```python
from build123d import *

# Parameters (mm, degrees)
SKETCH_1_W          = 20
SKETCH_1_H          = 12
SKETCH_1_W_2        = 4.2
SKETCH_1_H_2        = 6.9
EXTRUDE_1_DEPTH     = 9.5
CUT_EXTRUDE_START   = 9.5
SKETCH_1_4_W        = 20
SKETCH_1_4_H        = 3
CUT_EXTRUDE_2_DEPTH = 1
SKETCH_1_6_W        = 8.2
SKETCH_1_6_H        = 6.9
CUT_EXTRUDE_4_DEPTH = 2
SKETCH_2_R          = 0.7
SKETCH_2_R_2        = 0.35
CUT_EXTRUDE_5_DEPTH = 26.184320519
SKETCH_2_3_R        = 1
CUT_EXTRUDE_6_DEPTH = 7.5


with BuildPart() as part:
    # 草图1 → 凸台-拉伸1 (new body)
    with BuildSketch(Plane(origin=(0, 0, 0), x_dir=(1, 0, 0), z_dir=(0, 1, 0))):
        with Locations((10, -6)):
            Rectangle(SKETCH_1_W, SKETCH_1_H)
        with Locations((8, -8.25)):
            Rectangle(SKETCH_1_W_2, SKETCH_1_H_2, mode=Mode.SUBTRACT)
    extrude(amount=EXTRUDE_1_DEPTH)

    # 草图1<4> → 切除-拉伸2 (cut)
    with BuildSketch(Plane(origin=(0, 0, 0), x_dir=(1, 0, 0), z_dir=(0, 1, 0)).offset(CUT_EXTRUDE_START)):
        with Locations((10, -8)):
            Rectangle(SKETCH_1_4_W, SKETCH_1_4_H)
    extrude(amount=-CUT_EXTRUDE_2_DEPTH, mode=Mode.SUBTRACT)

    # 草图1<6> → 切除-拉伸4 (cut)
    with BuildSketch(Plane(origin=(0, 0, 0), x_dir=(1, 0, 0), z_dir=(0, 1, 0)).offset(CUT_EXTRUDE_START)):
        with Locations((8, -8.25)):
            Rectangle(SKETCH_1_6_W, SKETCH_1_6_H)
    extrude(amount=-CUT_EXTRUDE_4_DEPTH, mode=Mode.SUBTRACT)

    # 草图2 → 切除-拉伸5 (cut, through all)
    with BuildSketch(Plane(origin=(0, 9.5, 0), x_dir=(1, 0, 0), z_dir=(0, 1, 0))):
        with Locations(Location((3, -3, 0), (0, 0, 270))):
            Circle(SKETCH_2_R)
        with Locations(Location((3, -9, 0), (0, 0, 270))):
            Circle(SKETCH_2_R)
        with Locations(Location((17, -3, 0), (0, 0, 270))):
            Circle(SKETCH_2_R)
        with Locations(Location((17, -9, 0), (0, 0, 270))):
            Circle(SKETCH_2_R)
        with Locations(Location((7, -3, 0), (0, 0, 270))):
            Circle(SKETCH_2_R_2)
        with Locations(Location((14, -3, 0), (0, 0, 270))):
            Circle(SKETCH_2_R_2)
        with Locations(Location((3, -6, 0), (0, 0, 270))):
            Circle(SKETCH_2_R_2)
        with Locations(Location((17, -6, 0), (0, 0, 270))):
            Circle(SKETCH_2_R_2)
    extrude(amount=-CUT_EXTRUDE_5_DEPTH, mode=Mode.SUBTRACT)

    # 草图2<3> → 切除-拉伸6 (cut)
    with BuildSketch(Plane(origin=(0, 9.5, 0), x_dir=(1, 0, 0), z_dir=(0, 1, 0))):
        with Locations(Location((3, -3, 0), (0, 0, 270))):
            Circle(SKETCH_2_3_R)
        with Locations(Location((3, -9, 0), (0, 0, 330))):
            Circle(SKETCH_2_3_R)
        with Locations(Location((17, -3, 0), (0, 0, 270))):
            Circle(SKETCH_2_3_R)
        with Locations(Location((17, -9, 0), (0, 0, 330))):
            Circle(SKETCH_2_3_R)
    extrude(amount=-CUT_EXTRUDE_6_DEPTH, mode=Mode.SUBTRACT)


solid = part.part
```
Input: part model. Units: mm. Frame: model coordinates. A direction names the side the tool comes from. Coordinates: 2 decimals unless noted, no trailing zeros. Write each loop counter-clockwise with the first axis right and the second up, starting at its lowest first coordinate (ties: lowest second). Pieces come first, ordered by that corner, then holes.
1) Mould query, pull axis Z, two halves, no side actions, for faces 1 (the flat face through (10, 5, 12)), 2 (the flat face through (20, 5, 6)), 3 (the flat face through (1, 8.5, 8)). Classes: pulls with the +Z half, pulls with the -Z half, needs draft (parallel to the pull), parting line crosses it, or undercut.
2) Material intervals for line 1 along X through (y, z) = (0.8, 9); line 2 along X through (y, z) = (7.75, 9); line 3 along X through (y, z) = (7, 9), sorted ascending.
3) Section D-D on z = 9. Output: boundary loops of the cut face in (x, y), and give its area (3 significant figures).
4) Section A-A on z = 11.25. Output: boundary loops of the cut face in (x, y), and give its area (3 significant figures).
5) Pin query (flat end, axial travel): pin 1 Ø1.5 at (x, z) = (11.5, 7) entering from -Y; pin 2 Ø1 at (x, z) = (11, 6.5) entering from +Y. Return the tip coordinate at first contact, or that it passes through.
6) Set-up query: faces 4 (the flat face through (0, 5, 6)), 5 (the flat face through (10.1, 4, 8)), 6 (the flat face through (1, 9, 9.5)), 7 (the cylindrical face through (2.324, 5.802, 9.737)). Return all of +Z, -Z, +X, -X, +Y, -Y with unobstructed straight access to the full face (end or side cutting, diameter ignored); none if empty.
7) Section B-B on x = 6.25. Output: boundary loops of the cut face in (y, z).
8) Section C-C on y = 4.75. State how many separate pieces and enclosed holes the cut face has, and give its area (3 significant figures).
Check result:
1. face 1: pulls with the +Z half
1. face 2: needs draft
1. face 3: undercut
2. line 1: x = 0 to 2.3, 3.7 to 5.9, 10.1 to 16.3, 17.7 to 20
2. line 2: x = 0 to 2, 12.1 to 16, 18 to 20
2. line 3: x = 0 to 2, 4 to 5.9, 10.1 to 16, 18 to 20
3. outline: (0, 0) - (2.3, 0) - (2.3, 2) - (2, 2) - (2, 8.5) - (0, 8.5) - close; (3.7, 0) - (5.9, 0) - (5.9, 7.5) - (4, 7.5) - (4, 2) - (3.7, 2) - close; (10.1, 0) - (16.3, 0) - (16.3, 2) - (16, 2) - (16, 8.5) - (12.1, 8.5) - (12.1, 7.5) - (10.1, 7.5) - close; (17.7, 0) - (20, 0) - (20, 8.5) - (18, 8.5) - (18, 2) - (17.7, 2) - close
3. area: 98.8 mm2
4. outline: (0, 0) - (5.9, 0) - (5.9, 7.5) - (3.9, 7.5) - (3.9, 9.5) - (0, 9.5) - close; (10.1, 0) - (20, 0) - (20, 9.5) - (12.1, 9.5) - (12.1, 7.5) - (10.1, 7.5) - close
4. area: 142 mm2
5. pin 1: stops at y = 0
5. pin 2: stops at y = 7.5
6. face 4: +Z, -Z, -X, +Y, -Y
6. face 5: +Y, -Y
6. face 6: +X, -X, +Y
6. face 7: +Y
7. outline: (0, 0) - (9.5, 0) - (9.5, 4.8) - (0, 4.8) - close; (0, 11.7) - (9.5, 11.7) - (9.5, 12) - (0, 12) - close
8. separate pieces: 1
8. enclosed holes: 9
8. area: 197 mm2
